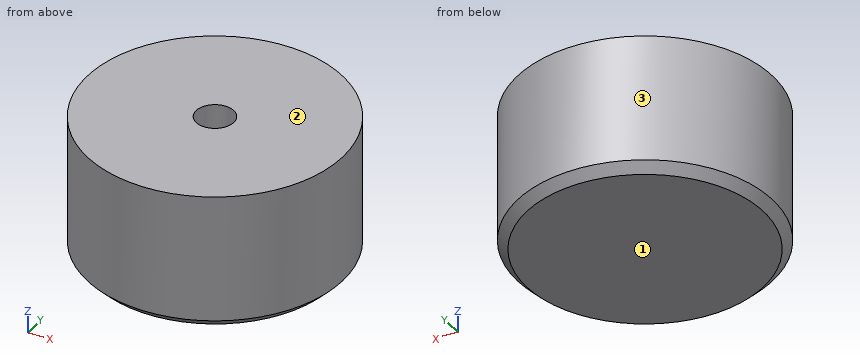
Autodesk Inventor part; units mm, degrees
ref_plane "YZ Plane" through (0, 0, 0) normal (1, 0, 0) x (0, 1, 0)
ref_plane "XZ Plane" through (0, 0, 0) normal (0, 1, 0) x (-1, 0, 0)
ref_plane "XY Plane" through (0, 0, 0) normal (0, 0, 1) x (1, 0, 0)
sketch "Skizze1" plane through (0, 0, 0) normal (0, 0, 1) x (1, 0, 0)
  line L0 (-19.6, 0) -> (19.6, 0)
  line L1 (0, -19.6) -> (0, 19.6)
  circle A0 centre (0, 0) radius 14
  dimension "d0" = 28
extrude "Extrusion1" add sketch "Skizze1" along normal blind 15
chamfer "Fase1" distance 1 angle 45 1 edges at (-14, 0, 0)
sketch "Skizze2" plane through (0, 0, 15) normal (0, 0, 1) x (1, 0, 0)
  point P0 (0, 0)
  point P1 (0, 0)
hole "Bohrung1" at (0, 0, 15) direction (0, 0, -1) diameter 4.134 depth 11 tip angle 118
properties part number "Gummistopl klein"
Work out the finished part from the listing and answer in its coordinate system (mm). Face numbers are marked on the shaded views. Give positions to 0.01 mm unless a question says otherwise; leave off trailing zeros. Order: outer loops, then holes, each group sorted by start corner. A loop starts at its lowest first (then second) coordinate and runs counter-clockwise, first axis right, second up. Notation, with made-up numbers: (61.5, 1.5) - (75.5, 1.5) arc R18 cw to (75.5, 12.5) - close; hole circle Ø1 at (0, -16.75). An arc over 180 degrees is marked (long way). One line per item, written item: value. Start each with the question number.
1. Each of these flat-tipped pins is pushed along its axis until it touches: pin 1 Ø6.5 at (x, y) = (0, 0) entering from -Z; pin 2 Ø1.5 at (x, z) = (-4.5, 11.5) entering from +Y; pin 3 Ø3 at (y, z) = (-6, 3.5) entering from -X; pin 4 Ø1 at (x, z) = (7.5, 12) entering from +Y. Where does it stop, or does it pass through?
2. Section A-A, the plane z = 8 is taken. Write down the section's boundary in (x, y), then the cut area to 3 significant figures.
3. Consider line 1 (Y direction, x = 0, z = 11.25); line 2 (Y direction, x = 1.25, z = 13). Determine where each line is inside the solid, lowest interval first.
4. For a pull along Z with two mould halves and no side action, classify the marked faces 1, 2 and 3 as released by +Z, released by -Z, zero draft, split by the parting line, or undercut.
Filled sheet:
1. pin 1: z = 0
1. pin 2: y = 13.49
1. pin 3: x = -13.26
1. pin 4: y = 12.12
2. outline: circle Ø28 at (0, 0); hole circle Ø4.13 at (0, 0)
2. area: 602 mm²
3. line 1: -14 to -2.07, 2.07 to 14
3. line 2: -13.94 to -1.65, 1.65 to 13.94
4. face 1: released by -Z
4. face 2: released by +Z
4. face 3: zero draft
